from build123d import *

# Parameters (mm, degrees)
PAD_DEPTH = 2
FILLET_R  = 2


with BuildPart() as part:
    # Sketch → Pad (new body)
    with BuildSketch(Plane.XY):
        with BuildLine():
            Line((-91.5, 56.984227), (-91.5, 8.434227))
            Line((-82, 8.434227), (-91.5, 8.434227))
            Line((-82, -12.265773), (-82, 8.434227))
            Line((-91.5, -12.265773), (-82, -12.265773))
            Line((-91.5, -12.265773), (-91.5, -51.515773))
            ThreePointArc((-91.5, -51.515773), (-89.522971, -56.288744), (-84.75, -58.265773))
            Line((-84.75, -58.265773), (-59.8, -58.265773))
            Line((-59.8, -48.765773), (-59.8, -58.265773))
            Line((-39.1, -48.765773), (-59.8, -48.765773))
            Line((-39.1, -58.265773), (-39.1, -48.765773))
            Line((-39.1, -58.265773), (39.1, -58.265773))
            Line((39.1, -48.765773), (39.1, -58.265773))
            Line((59.8, -48.765773), (39.1, -48.765773))
            Line((59.8, -58.265773), (59.8, -48.765773))
            Line((59.8, -58.265773), (84.75, -58.265773))
            ThreePointArc((84.75, -58.265773), (89.522971, -56.288744), (91.5, -51.515773))
            Line((91.5, -51.515773), (91.5, -12.265773))
            Line((82, -12.265773), (91.5, -12.265773))
            Line((82, 8.434227), (82, -12.265773))
            Line((91.5, 8.434227), (82, 8.434227))
            Line((91.5, 8.434227), (91.5, 56.984227))
            ThreePointArc((91.5, 56.984227), (89.522971, 61.757197), (84.75, 63.734227))
            Line((84.75, 63.734227), (-84.75, 63.734227))
            ThreePointArc((-84.75, 63.734227), (-89.522971, 61.757197), (-91.5, 56.984227))
        make_face()
    extrude(amount=PAD_DEPTH)

    # Fillet
    fillet_edges = [part.edges().sort_by_distance(p)[0] for p in [
        (-82, 8.434227, 1),
        (-91.5, 8.434227, 1),
        (-82, -12.265773, 1),
        (-91.5, -12.265773, 1),
        (-39.1, -48.765773, 1),
        (-59.8, -48.765773, 1),
        (39.1, -48.765773, 1),
        (-59.8, -58.265773, 1),
        (-39.1, -58.265773, 1),
        (39.1, -58.265773, 1),
        (59.8, -48.765773, 1),
        (59.8, -58.265773, 1),
        (82, 8.434227, 1),
        (91.5, 8.434227, 1),
        (91.5, -12.265773, 1),
        (82, -12.265773, 1),
    ]]
    fillet(fillet_edges, radius=FILLET_R)


solid = part.part
CAD build for the part. Positions are in the model's coordinates, mm. Give positions to 0.01 mm unless a question says otherwise; leave off trailing zeros. Write each loop counter-clockwise with the first axis right and the second up, starting at its lowest first coordinate (ties: lowest second). Pieces come first, ordered by that corner, then holes. Notation, with made-up numbers: M 32,-5 L 78,-5 A19 cw 78,11 Z; hole C -25,-23.75 d6. An arc over 180 degrees is marked long. Put each result on its own line as item: value. Start each with the question number.
(1) Band-saw the part on A-A, the plane x = -50. Write the cut outline in (y, z).
(2) Band-saw the part on B-B, the plane y = -5. Write the cut outline in (x, z).
(3) Flat gauge pins, fed straight in: pin 1 Ø0.6 at (y, z) = (-6, 1) entering from -X; pin 2 Ø0.6 at (x, z) = (86, 1) entering from +Y; pin 3 Ø1 at (x, z) = (-50, 1) entering from -Y. Where does each tip first touch, or does it go through?
(4) Probe L1, parallel to X at y = -6, z = 0.85; L2, parallel to Y at x = 52.5, z = 1.2. List the from-to ranges inside material, lowest first.
Response values:
1. outline: M -48.77,0 L 63.73,0 L 63.73,2 L -48.77,2 Z
2. outline: M -82,0 L 82,0 L 82,2 L -82,2 Z
3. pin 1: stops at x = -82
3. pin 2: stops at y = 63.67
3. pin 3: stops at y = -48.77
4. L1: x = -82 to 82
4. L2: y = -48.77 to 63.73
